from build123d import *

# Parameters (mm, degrees)
SKETCH1_W           = 165
SKETCH1_H           = 100
BOSS_EXTRUDE1_DEPTH = 8
SKETCH1_4_R         = 1.75
SKETCH1_4_R_2       = 1.742752204
SKETCH1_4_W         = 165
SKETCH1_4_H         = 100
BOSS_EXTRUDE2_DEPTH = 3
FILLET3_R           = 3.5


with BuildPart() as part:
    # Sketch1 → Boss-Extrude1 (new body)
    with BuildSketch(Plane.XY):
        with Locations((88.5, 63.5)):
            Rectangle(SKETCH1_W, SKETCH1_H)
    extrude(amount=BOSS_EXTRUDE1_DEPTH)

    # Sketch1<4> → Boss-Extrude2 (add)
    with BuildSketch(Plane.XY):
        Polygon((7, 122), (7, 118), (165, 118), (165, 122), (172, 122), (172, 0), (165, 0), (165, 4), (56, 4), (56, 0), (49, 0), (49, 4), (7, 4), (7, 0), (0, 0), (0, 122), align=None)
        with Locations((3.5, 118.5)):
            Circle(SKETCH1_4_R, mode=Mode.SUBTRACT)
        with Locations((168.5, 118.5)):
            Circle(SKETCH1_4_R, mode=Mode.SUBTRACT)
        with Locations((168.5, 3.5)):
            Circle(SKETCH1_4_R, mode=Mode.SUBTRACT)
        with Locations((3.5, 3.5)):
            Circle(SKETCH1_4_R, mode=Mode.SUBTRACT)
        with Locations((52.5, 3.5)):
            Circle(SKETCH1_4_R, mode=Mode.SUBTRACT)
        with Locations((3.5, 61.5)):
            Circle(SKETCH1_4_R_2, mode=Mode.SUBTRACT)
        with Locations((88.5, 63.5)):
            Rectangle(SKETCH1_4_W, SKETCH1_4_H, mode=Mode.SUBTRACT)
    extrude(amount=BOSS_EXTRUDE2_DEPTH)

    # Fillet3
    fillet3_edges = [part.edges().sort_by_distance(p)[0] for p in [
        (56, 0, 1.5),
        (165, 0, 1.5),
        (172, 0, 1.5),
        (49, 0, 1.5),
        (0, 0, 1.5),
        (7, 0, 1.5),
        (0, 122, 1.5),
        (7, 122, 1.5),
        (172, 122, 1.5),
        (165, 122, 1.5),
    ]]
    fillet(fillet3_edges, radius=FILLET3_R - 0.0001)  # a hair under: the kernel refuses the full size


solid = part.part
Can you work these out from the model? Positions are in its coordinate system, mm. A direction names the side the tool comes from. Coordinates: 2 decimals unless noted, no trailing zeros. Loops run counter-clockwise (first coordinate to the right, second up) from the corner with the lowest first, then second, coordinate; pieces in that order, holes last. Notation, with made-up numbers: (-22.5, 27.25) - (-10.5, 27.25) arc R14 ccw to (-10.5, 46.25) - close; hole circle Ø2 at (-3, 72). An arc over 180 degrees is marked (long way). Answer as a JSON object with one key per item and string values. Group by question number.
Item 1: If we section it at D-D (z = 5.5): List the corners of the cut face in (x, y) for me.
Item 2: If we mould it in two halves opening along X, with no side actions, what happens to faces 1 (the face through (87, 13.5, 5)), 2 (the face through (166.05, 1, 1.52)), 3 (the face through (171, 63, 5)), 4 (the face through (6, 63, 5))? For each: released by +X, released by -X, zero draft, split by the parting line, or undercut.
Item 3: If we section it at C-C (y = 23): List the corners of the cut face in (x, z) for me, plus the area to 3 significant figures.
Item 4: If I drill on L1, parallel to X at y = 118.5, z = 1.8; L2, parallel to Y at x = 3.5, z = 2; L3, parallel to X at y = 78.5, z = 3.25, over which ranges is the centre line in solid material (lowest first)? Write a range as from..to.
Item 5: For pin 1 (4.5 mm diameter, centred on x = 168.5, y = 3.5, fed in from +Z); pin 2 (1 mm diameter, centred on y = 13.5, z = 6.5, fed in from -X); pin 3 (2.5 mm diameter, centred on x = 103, z = 2, fed in from -Y); pin 4 (3 mm diameter, centred on x = 3.5, y = 61.5, fed in from -Z), each with a flat end and sliding along its axis, tell me the tip position at first contact or that it passes through.
Item 6: If we section it at A-A (y = 61.5): List the corners of the cut face in (x, z) for me, plus the area to 3 significant figures.
Item 7: If we section it at B-B (x = 141.5): List the corners of the cut face in (y, z) for me.
Item 8: On a 3-axis mill with a long thin cutter (end or side, diameter ignored), from which of +Z, -Z, +X, -X, +Y, -Y can I reach the whole of each face in a straight line? I mean faces 5 (the face through (50, 1.05, 1.52)), 6 (the face through (6, 120.95, 1.52)), 7 (the face through (170.169, 4.026, 1.479)). Say none if no direction works.
Returned:
{
 "1": {"outline": "(6, 13.5) - (171, 13.5) - (171, 113.5) - (6, 113.5) - close"},
 "2": {"face 1": "zero draft", "face 2": "undercut", "face 3": "released by +X", "face 4": "released by -X"},
 "3": {"outline": "(0, 0) - (172, 0) - (172, 3) - (171, 3) - (171, 8) - (6, 8) - (6, 3) - (0, 3) - close", "area": "1,340 mm²"},
 "4": {"L1": "x = 0..1.75, 5.25..7, 165..166.75, 170.25..172", "L2": "y = 0..1.75, 5.25..59.76, 63.24..116.75, 120.25..122", "L3": "x = 6..171"},
 "5": {"pin 1": "stops at z = 3", "pin 2": "stops at x = 6", "pin 3": "stops at y = 4", "pin 4": "passes through"},
 "6": {"outline": "(0, 0) - (1.76, 0) - (1.76, 3) - (0, 3) - close; (5.24, 0) - (172, 0) - (172, 3) - (171, 3) - (171, 8) - (6, 8) - (6, 3) - (5.24, 3) - close", "area": "1,330 mm²"},
 "7": {"outline": "(4, 0) - (118, 0) - (118, 3) - (113.5, 3) - (113.5, 8) - (13.5, 8) - (13.5, 3) - (4, 3) - close"},
 "8": {"face 5": "+Z, -Z, -Y", "face 6": "+Z, -Z, +Y", "face 7": "+Z, -Z"}
}
